Source: CAD feature listing. Evaluate the final solid. Frame: model axes, mm. Face numbers are marked on the shaded views. A direction names the side the tool comes from. Give positions to 0.01 mm unless a question says otherwise; leave off trailing zeros. Order: outer loops, then holes, each group sorted by start corner. A loop starts at its lowest first (then second) coordinate and runs counter-clockwise, first axis right, second up. Notation, with made-up numbers: M -26.5,81 L 26.5,81 A11 ccw 26.5,99 Z; hole C -21.5,20 d11. An arc over 180 degrees is marked long. Answer as a JSON object with one key per item and string values. Group by question number.
1. Material intervals for L1, parallel to X at y = 5.5, z = -31.5; L2, parallel to Y at x = -20, z = -43.85, sorted ascending. Write a range as [from, to].
2. Pin query (flat end, axial travel): P1, Ø3.5, axis at x = -35, y = 87, coming from the +Z side; P2, Ø12.5, axis at x = -17, z = -28.5, coming from the +Y side. Return the tip coordinate at first contact, or that it passes through.
3. Section query A-A (y = 87). Count the separate pieces of the cut face and the enclosed holes in it, plus the area to 3 significant figures.
4. Section query B-B (x = -20). Output: boundary loops of the cut face in (y, z), plus the area to 3 significant figures.
5. Pull-direction query (Z, two-part tool) for the marked faces 1, 2 and 3; classes: +Z half, -Z half, draft (parallel to the pull), parting line (faces both ways), or undercut.
6. Set-up query: the marked faces 4 and 5. Return all of +Z, -Z, +X, -X, +Y, -Y with unobstructed straight access to the full face (end or side cutting, diameter ignored); none if empty.
7. Section query C-C (z = -38). Output: boundary loops of the cut face in (x, y).
8. Section query D-D (y = 47). Output: boundary loops of the cut face in (x, z), plus the area to 3 significant figures.
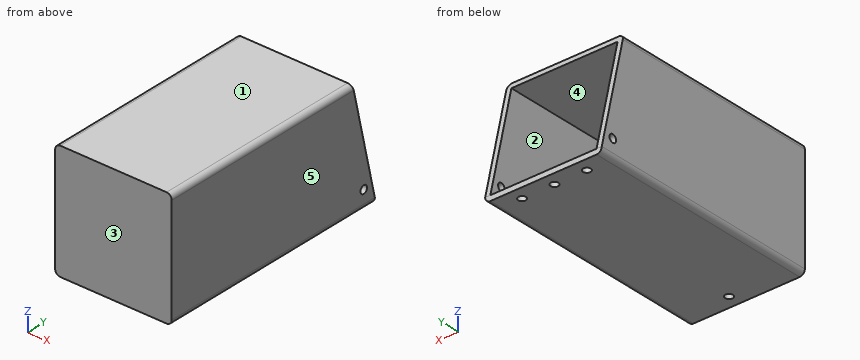
Autodesk Inventor part; units mm, degrees
ref_plane "YZ Plane" through (0, 0, 0) normal (1, 0, 0) x (0, 1, 0)
ref_plane "XZ Plane" through (0, 0, 0) normal (0, 1, 0) x (-1, 0, 0)
ref_plane "XY Plane" through (0, 0, 0) normal (0, 0, 1) x (1, 0, 0)
sketch "Sketch1" plane through (0, 0, 0) normal (0, 1, 0) x (-1, 0, 0)
  line L0 (0, 0) -> (45, 0)
  line L1 (45, 0) -> (45, -45)
  line L2 (45, -45) -> (0, -45)
  line L3 (0, -45) -> (0, 0)
  dimension "d0" = 45
  dimension "d1" = 45
extrude "Extrusion1" add sketch "Sketch1" along normal blind 2
sketch "Sketch2" plane through (0, 2, 0) normal (0, 1, 0) x (1, 0, 0)
  line L0 (-45, 0) -> (0, 0)
  line L1 (-22.5, 0) -> (-22.5, 45)
  line L2 (0, 45) -> (-45, 45)
  line L3 (0, 0) -> (0, 45)
  line L4 (0, 22.5) -> (-45, 22.5)
  line L5 (-45, 45) -> (-45, 0)
  line L6 (-43, 2) -> (-2, 2)
  line L7 (-2, 2) -> (-2, 43)
  line L8 (-2, 43) -> (-43, 43)
  line L9 (-43, 43) -> (-43, 2)
  point P0 (-43, 22.5)
  point P1 (-22.5, 43)
  dimension "d10" = 3
  dimension "d4" = 41
  dimension "d5" = 41
extrude "Extrusion2" add sketch "Sketch2" along normal blind 90 contours L5 L4 L9 L6 L1 L0 | L1 L6 L7 L4 L3 L0 | L5 L2 L1 L8 L9 L4 | L4 L7 L8 L1 L2 L3
sketch "Sketch3" plane through (0, 0, -45) normal (0, 0, -1) x (-1, 0, 0)
  line L0 (45, 0) -> (45, 92)
  line L1 (45, 0) -> (20, 0)
  line L2 (20, 0) -> (20, 5)
  line L3 (20, 5) -> (45, 5)
  line L4 (45, 5) -> (45, 0)
  circle A0 centre (20, 5) radius 1.5
  point P0 (0, 0)
  dimension "d8" = 25
  dimension "d9" = 5
  dimension "d10" = 3
extrude "Extrusion3" cut sketch "Sketch3" against normal blind 5 contours A0 L2 L3 | L3 L2 A0
fillet "Fillet1" radius 2 4 edges at (0, 46, -45) (-45, 46, -45) (-45, 46, 0) (0, 46, 0)
sketch "Sketch5" plane through (-43, 2, -43) normal (0, 0, 1) x (1, 0, 0)
  line L0 (0, 90) -> (41, 90)
  line L1 (-2, 80) -> (20.5, 80)
  line L2 (20.5, 80) -> (20.5, 85)
  line L3 (20.5, 85) -> (-2, 85)
  line L4 (-2, 85) -> (-2, 80)
  line L5 (-2, 80) -> (8, 80)
  line L6 (8, 80) -> (8, 85)
  line L7 (8, 85) -> (-2, 85)
  line L8 (-2, 85) -> (-2, 80)
  line L9 (0, 90) -> (41, 90)
  line L10 (43, 80) -> (33, 80)
  line L11 (33, 80) -> (33, 85)
  line L12 (33, 85) -> (43, 85)
  line L13 (43, 85) -> (43, 80)
  circle A0 centre (8, 85) radius 1.5
  circle A1 centre (20.5, 85) radius 1.5
  circle A2 centre (33, 85) radius 1.5
  point P0 (43, -2)
  dimension "d19" = 22.5
  dimension "d20" = 5
  dimension "d21" = 10
  dimension "d22" = 5
  dimension "d23" = 10
  dimension "d24" = 5
  dimension "d25" = 3
  dimension "d26" = 3
  dimension "d27" = 3
extrude "Extrusion5" cut sketch "Sketch5" against normal blind 10 contours A0 L3 L6 | L6 L3 A0 | A0 L3 | A1 L3 L2 | L2 L3 A1 | A2 L12 L11 | L11 L12 A2
sketch "Sketch6" plane through (0, 0, -2) normal (1, 0, 0) x (0, 0, -1)
  line L0 (41, 92) -> (41, 0)
  line L1 (-2, 0) -> (-2, 92)
  line L2 (41, 92) -> (-2, 92)
  line L3 (-2, 92) -> (-2, 82)
  line L4 (-2, 82) -> (41, 92)
  dimension "d30" = 10
extrude "Extrusion6" cut sketch "Sketch6" against normal blind 90
sketch "Sketch7" plane through (-45, 0, -43) normal (-1, 0, 0) x (0, 0, 1)
  line L0 (0, 2) -> (0, 92)
  line L1 (0, 92) -> (5, 92)
  line L2 (5, 92) -> (5, 87)
  line L3 (5, 87) -> (0, 87)
  line L4 (0, 87) -> (0, 92)
  circle A0 centre (5, 87) radius 1.5
  point P0 (43, 0)
  dimension "d33" = 5
  dimension "d34" = 5
  dimension "d35" = 3
extrude "Extrusion7" cut sketch "Sketch7" against normal blind 90 contours A0 L2 L3 | L3 L2 A0
properties part number "reduced_turtle"
Answer sheet:
{
 "1": {"L1": "[-45, -43], [-2, 0]", "L2": "[0, 3.5], [6.5, 92]"},
 "2": {"P1": "z = -43", "P2": "y = 2"},
 "3": {"separate pieces": "6", "enclosed holes": "0", "area": "144 mm^2"},
 "4": {"outline": "M 0,-45 L 3.5,-45 L 3.5,-43 L 2,-43 L 2,-2 L 82.47,-2 L 82,0 L 0,0 Z; M 6.5,-45 L 92,-45 L 92,-43 L 6.5,-43 Z", "area": "424 mm^2"},
 "5": {"face 1": "+Z half", "face 2": "undercut", "face 3": "draft"},
 "6": {"face 4": "+Y", "face 5": "+Z, -Z, +X, +Y, -Y"},
 "7": {"outline": "M -45,0 L 0,0 L 0,85.5 L -2,85.5 L -2,2 L -43,2 L -43,85.5 L -45,85.5 Z; M -45,88.5 L -43,88.5 L -43,90.84 L -45,90.84 Z; M -2,88.5 L 0,88.5 L 0,90.84 L -2,90.84 Z"},
 "8": {"outline": "M -45,-43 A2 ccw -43,-45 L -2,-45 A2 ccw 0,-43 L 0,-2 A2 ccw -2,0 L -43,0 A2 ccw -45,-2 Z; hole M -43,-43 L -2,-43 L -2,-2 L -43,-2 Z", "area": "341 mm^2"}
}
